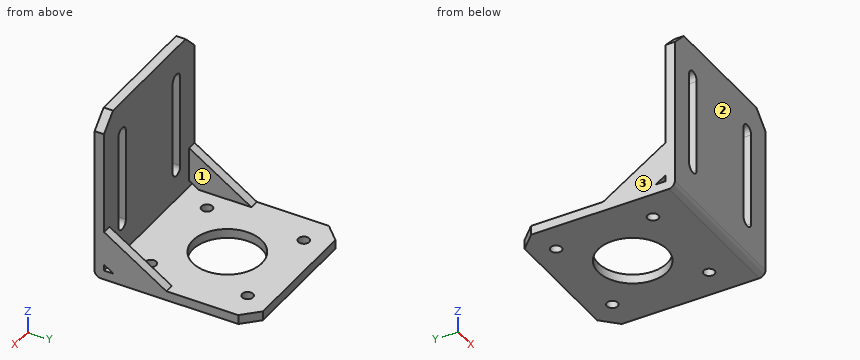
```python
from build123d import *

# Parameters (mm, degrees)
SKETCH_1_R          = 1.75
SKETCH_1_R_2        = 11.05
EXTRUDE_1_DEPTH     = 3
SKETCH_2_W          = 50
SKETCH_2_H          = 3
EXTRUDE_2_DEPTH     = 51
FILLET_1_R          = 2
CUT_EXTRUDE_1_DEPTH = 51
CHAMFER_1_SIZE      = 5
EXTRUDE_3_DEPTH     = 3
FILLET_3_R          = 2


with BuildPart() as part:
    # 草图1 → 凸台-拉伸1 (new body)
    with BuildSketch(Plane.XY):
        Polygon((25, 29.708680022), (25, -16.291319978), (-25, -16.291319978), (-25, 29.708680022), (-20, 34.708680022), (20, 34.708680022), align=None)
        with Locations((-15.5, 27.208680022)):
            Circle(SKETCH_1_R, mode=Mode.SUBTRACT)
        with Locations((15.5, 27.208680022)):
            Circle(SKETCH_1_R, mode=Mode.SUBTRACT)
        with Locations((-15.5, -3.791319978)):
            Circle(SKETCH_1_R, mode=Mode.SUBTRACT)
        with Locations((15.5, -3.791319978)):
            Circle(SKETCH_1_R, mode=Mode.SUBTRACT)
        with Locations((0, 11.708680022)):
            Circle(SKETCH_1_R_2, mode=Mode.SUBTRACT)
    extrude_1 = extrude(amount=EXTRUDE_1_DEPTH)

    # 草图2 → 凸台-拉伸2 (add)
    with BuildSketch(Plane.XY.offset(3)):
        with Locations((0, -14.791319978)):
            Rectangle(SKETCH_2_W, SKETCH_2_H)
    extrude(amount=EXTRUDE_2_DEPTH)

    # 圆角1
    fillet_1_edges = [part.edges().sort_by_distance(p)[0] for p in [
        (0, -16.291319978, 0),
    ]]
    fillet(fillet_1_edges, radius=FILLET_1_R)

    # 草图3 → 切除-拉伸1 (cut)
    with BuildSketch(Plane(origin=(0, -13.291319978, 0), x_dir=(1, 0, 0), z_dir=(0, 1, 0))):
        with BuildLine():
            Line((-17.1, -13), (-17.1, -43))
            ThreePointArc((-17.1, -43), (-15, -45.1), (-12.9, -43))
            Line((-12.9, -43), (-12.9, -13))
            ThreePointArc((-12.9, -13), (-15, -10.9), (-17.1, -13))
        make_face()
        with BuildLine():
            Line((12.9, -13), (12.9, -43))
            ThreePointArc((12.9, -43), (15, -45.1), (17.1, -43))
            Line((17.1, -43), (17.1, -13))
            ThreePointArc((17.1, -13), (15, -10.9), (12.9, -13))
        make_face()
    extrude(amount=-CUT_EXTRUDE_1_DEPTH, mode=Mode.SUBTRACT)

    # 倒角1
    chamfer_1_edges = [part.edges().sort_by_distance(p)[0] for p in [
        (-25, -14.791319978, 54),
        (25, -14.791319978, 54),
    ]]
    chamfer(chamfer_1_edges, length=CHAMFER_1_SIZE)

    # 草图4 → 凸台-拉伸3 (add)
    with BuildSketch(Plane(origin=(25, 0, 0), x_dir=(0, 0, -1), z_dir=(1, 0, 0))):
        Polygon((-3, 6.708680022), (-16, -13.291319978), (-5, -13.291319978), (-3, -10.214396901), align=None)
    extrude_3 = extrude(amount=-EXTRUDE_3_DEPTH)

    # 镜向1: 凸台-拉伸1, 凸台-拉伸3 across plane
    add(extrude_1.mirror(Plane(origin=(0, 0, 0), x_dir=(0, 0, 1), z_dir=(1, 0, 0))))
    add(extrude_3.mirror(Plane(origin=(0, 0, 0), x_dir=(0, 0, 1), z_dir=(1, 0, 0))))

    # 圆角3
    fillet_3_edges = [part.edges().sort_by_distance(p)[0] for p in [
        (0, -16.291319978, 0),
    ]]
    fillet(fillet_3_edges, radius=FILLET_3_R)


solid = part.part
```
Can you work these out from the model? Positions are in its coordinate system, mm. Face numbers are marked on the shaded views. Round coordinates to 2 decimals unless told otherwise and drop trailing zeros. Order: outer loops, then holes, each group sorted by start corner. A loop starts at its lowest first (then second) coordinate and runs counter-clockwise, first axis right, second up. Notation, with made-up numbers: (51.5, 40) -> (110.5, 40) arc R22 ccw to (110.5, 67) -> close; hole circle Ø4 at (3.5, 43). An arc over 180 degrees is marked (long way). Return JSON: item names as keys, results as strings. Group by question number.
1. If we section it at B-B, the plane x = -19: Write out the boundary of the cut face in (y, z).
2. Will these pins go through, and if not, where does the flat tip stop? pin 1 (3 mm diameter, centred on x = 20, z = 18, fed in from +Y); pin 2 (5 mm diameter, centred on x = 8, y = 14.5, fed in from -Z); pin 3 (5.5 mm diameter, centred on x = -15.5, y = -3.79, fed in from +Z).
3. If we section it at A-A, the plane z = 41: Write out the boundary of the cut face in (x, y), then the cut area to 3 significant figures.
4. If we section it at C-C, the plane y = 28: Write out the boundary of the cut face in (x, z).
5. If we section it at D-D, the plane x = -4: Write out the boundary of the cut face in (y, z).
6. We'd pull the mould along X, two halves only. Please class the marked faces 1, 2 and 3: released by +X, released by -X, zero draft, split by the parting line, or undercut.
7. I need wall thicknesses on line 1 (Y direction, x = -15.5, z = 2.1); line 2 (Y direction, x = -15, z = 1); line 3 (Z direction, x = 11.5, y = 2). Which ranges of each line are inside material? Lowest first, please. Write a range as [from, to].
Output values:
{
 "1": {"outline": "(-16.29, 2) arc R2 ccw to (-14.29, 0) -> (34.71, 0) -> (34.71, 3) -> (-13.29, 3) -> (-13.29, 54) -> (-16.29, 54) -> close"},
 "2": {"pin 1": "y = -13.29", "pin 2": "through", "pin 3": "z = 3"},
 "3": {"outline": "(-25, -16.29) -> (-17.1, -16.29) -> (-17.1, -13.29) -> (-25, -13.29) -> close; (-12.9, -16.29) -> (12.9, -16.29) -> (12.9, -13.29) -> (-12.9, -13.29) -> close; (17.1, -16.29) -> (25, -16.29) -> (25, -13.29) -> (17.1, -13.29) -> close", "area": "125 mm²"},
 "4": {"outline": "(-25, 0) -> (-17.06, 0) -> (-17.06, 3) -> (-25, 3) -> close; (-13.94, 0) -> (13.94, 0) -> (13.94, 3) -> (-13.94, 3) -> close; (17.06, 0) -> (25, 0) -> (25, 3) -> (17.06, 3) -> close"},
 "5": {"outline": "(-16.29, 2) arc R2 ccw to (-14.29, 0) -> (1.41, 0) -> (1.41, 3) -> (-13.29, 3) -> (-13.29, 54) -> (-16.29, 54) -> close; (22.01, 0) -> (34.71, 0) -> (34.71, 3) -> (22.01, 3) -> close"},
 "6": {"face 1": "undercut", "face 2": "zero draft", "face 3": "released by -X"},
 "7": {"line 1": "[-16.29, -5.54], [-2.04, 25.46], [28.96, 34.71]", "line 2": "[-16.02, -5.47], [-2.11, 25.53], [28.89, 34.71]", "line 3": "[0, 3]"}
}
